Could you check a few things on this model? Use its own coordinates, in mm. A direction names the side the tool comes from. Round coordinates to 2 decimals unless told otherwise and drop trailing zeros. Loops run counter-clockwise (first coordinate to the right, second up) from the corner with the lowest first, then second, coordinate; pieces in that order, holes last. Notation, with made-up numbers: (58, 9.5) -> (73, 9.5) arc R26 ccw to (73, 43.5) -> close; hole circle Ø3 at (68.5, 48.5). An arc over 180 degrees is marked (long way). Write each question's results on one line, items separated by ' | '.
from build123d import *

# Parameters (mm, degrees)
BOSS_EXTRUDE2_DEPTH = 15
SKETCH4_R           = 2
CUT_EXTRUDE1_DEPTH  = 1
SKETCH5_R           = 1.5
BOSS_EXTRUDE3_DEPTH = 0.5
SKETCH7_W           = 3
SKETCH7_H           = 3.5
CUT_EXTRUDE2_DEPTH  = 6
LPATTERN1_COUNT     = 3
LPATTERN1_PITCH     = 5.08
SKETCH8_W           = 1
SKETCH8_H           = 6.7
BOSS_EXTRUDE4_DEPTH = 0.8
SKETCH9_W           = 1
SKETCH9_H           = 6.7
CUT_EXTRUDE3_DEPTH  = 0.8


with BuildPart() as part:
    # Sketch3 → Boss-Extrude2 (new body)
    with BuildSketch(Plane(origin=(0, 0, 0), x_dir=(0, 0, -1), z_dir=(1, 0, 0))):
        with BuildLine():
            Line((-5.15, 0), (5.15, 0))
            Line((5.15, 0), (5.15, 5.1))
            Line((5.15, 5.1), (2.75, 14.1))
            Line((2.75, 14.1), (-3.35, 14.1))
            Line((-3.35, 14.1), (-4.15, 7.7))
            ThreePointArc((-4.15, 7.7), (-4.857106781, 7.407106781), (-5.15, 6.7))
            Line((-5.15, 6.7), (-5.15, 0))
        make_face()
    extrude(amount=BOSS_EXTRUDE2_DEPTH)

    # Sketch4 → Cut-Extrude1 (cut)
    with BuildSketch(Plane(origin=(0, 14.1, 0), x_dir=(1, 0, 0), z_dir=(0, 1, 0))):
        with Locations(Location((7.5, -0.3, 0), (0, 0, 270))):
            Circle(SKETCH4_R)
    cut_extrude1 = extrude(amount=-CUT_EXTRUDE1_DEPTH, mode=Mode.SUBTRACT)

    # Sketch5 → Boss-Extrude3 (add)
    with BuildSketch(Plane(origin=(0, 13.1, 0), x_dir=(1, 0, 0), z_dir=(0, 1, 0))):
        with Locations(Location((7.5, -0.3, 0), (0, 0, 270))):
            Circle(SKETCH5_R)
    boss_extrude3 = extrude(amount=BOSS_EXTRUDE3_DEPTH)

    # Sketch-Pattern1: Cut-Extrude1, Boss-Extrude3 at 2 more places
    with Locations((5.08, 0, 0), (-5.08, 0, 0)):
        add(cut_extrude1, mode=Mode.SUBTRACT)
        add(boss_extrude3)

    # Sketch7 → Cut-Extrude2 (cut)
    with BuildSketch(Plane.XY.offset(5.15)):
        with Locations((12.58, 3.35)):
            Rectangle(SKETCH7_W, SKETCH7_H)
    cut_extrude2 = extrude(amount=-CUT_EXTRUDE2_DEPTH, mode=Mode.SUBTRACT)

    # LPattern1: Cut-Extrude2 ×3
    with Locations(*[(-i * LPATTERN1_PITCH, 0, 0) for i in range(1, LPATTERN1_COUNT)]):
        add(cut_extrude2, mode=Mode.SUBTRACT)

    # Sketch8 → Boss-Extrude4 (add)
    with BuildSketch(Plane.ZY):
        with Locations((3.65, 3.35)):
            Rectangle(SKETCH8_W, SKETCH8_H)
        with Locations((-3.15, 3.35)):
            Rectangle(SKETCH8_W, SKETCH8_H)
    extrude(amount=BOSS_EXTRUDE4_DEPTH)

    # Sketch9 → Cut-Extrude3 (cut)
    with BuildSketch(Plane(origin=(15, 0, 0), x_dir=(0, 0, -1), z_dir=(1, 0, 0))):
        with Locations((3.15, 3.35)):
            Rectangle(SKETCH9_W, SKETCH9_H)
        with Locations((-3.65, 3.35)):
            Rectangle(SKETCH9_W, SKETCH9_H)
    extrude(amount=-CUT_EXTRUDE3_DEPTH, mode=Mode.SUBTRACT)


solid = part.part
1) I'm going to push flat-ended pins straight in: pin 1 (1.2 mm diameter, centred on x = 2, z = 0.5, fed in from +Y); pin 2 (5 mm diameter, centred on x = 10.5, y = 9.5, fed in from -Z); pin 3 (3 mm diameter, centred on y = 6, z = 1.5, fed in from -X). Where does each tip first touch, or does it pass through?
Model answer:
pin 1: stops at y = 13.6 | pin 2: stops at z = -4.64 | pin 3: stops at x = 0
2) I want a section at B-B, the plane x = 2.42. Write out the boundary of the cut face in (y, z).
Model answer:
outline: (0, -5.15) -> (5.1, -5.15) -> (14.1, -2.75) -> (14.1, -1.7) -> (13.1, -1.7) -> (13.1, -1.2) -> (13.6, -1.2) -> (13.6, 1.8) -> (13.1, 1.8) -> (13.1, 2.3) -> (14.1, 2.3) -> (14.1, 3.35) -> (7.7, 4.15) arc R1 ccw to (6.7, 5.15) -> (5.1, 5.15) -> (5.1, -0.85) -> (1.6, -0.85) -> (1.6, 5.15) -> (0, 5.15) -> close
3) For faces 1 (the flat face through (7, 14.1, -2)), 2 (the flat face through (14.6, 3.3, 4.15)), 3 (the cylindrical face through (14.067, 13.346, 0.105)), 4 (the flat face through (3.92, 3, 2)), which set-ups out of +Z, -Z, +X, -X, +Y, -Y let a thin tool reach every point of the face, with its end or its side?
Model answer:
face 1: +Z, -Z, +X, -X, +Y | face 2: +X, -Y | face 3: +Y | face 4: +Z
4) I need wall thicknesses on line 1 (X direction, y = 13.95, z = 0.3); line 2 (X direction, y = 1.75, z = -0.25); line 3 (Z direction, x = 14.5, y = 4.5). Which ranges of each line are inside material? Lowest first, please.
Model answer:
line 1: x = 0 to 0.42, 4.42 to 5.5, 9.5 to 10.58, 14.58 to 15 | line 2: x = 0 to 0.92, 3.92 to 6, 9 to 11.08, 14.08 to 15 | line 3: z = -5.15 to -3.65, -2.65 to 3.15, 4.15 to 5.15
5) I want a section at A-A, the plane z = 3.75. Write out the boundary of the cut face in (x, y).
Model answer:
outline: (-0.8, 0) -> (14.2, 0) -> (14.2, 6.7) -> (15, 6.7) -> (15, 10.9) -> (0, 10.9) -> (0, 6.7) -> (-0.8, 6.7) -> close; hole (0.92, 1.6) -> (3.92, 1.6) -> (3.92, 5.1) -> (0.92, 5.1) -> close; hole (6, 1.6) -> (9, 1.6) -> (9, 5.1) -> (6, 5.1) -> close; hole (11.08, 1.6) -> (14.08, 1.6) -> (14.08, 5.1) -> (11.08, 5.1) -> close
6) I want a section at C-C, the plane y = 6.25. Write out the boundary of the cut face in (x, z).
Model answer:
outline: (-0.8, -3.65) -> (0, -3.65) -> (0, -4.84) -> (15, -4.84) -> (15, -3.65) -> (14.2, -3.65) -> (14.2, -2.65) -> (15, -2.65) -> (15, 3.15) -> (14.2, 3.15) -> (14.2, 4.15) -> (15, 4.15) -> (15, 5.15) -> (0, 5.15) -> (0, 4.15) -> (-0.8, 4.15) -> (-0.8, 3.15) -> (0, 3.15) -> (0, -2.65) -> (-0.8, -2.65) -> close
7) I want a section at D-D, the plane x = 5.25. Write out the boundary of the cut face in (y, z), plus the area to 3 significant figures.
Model answer:
outline: (0, -5.15) -> (5.1, -5.15) -> (14.1, -2.75) -> (14.1, 3.35) -> (7.7, 4.15) arc R1 ccw to (6.7, 5.15) -> (0, 5.15) -> close | area: 125 mm2
8) If we mould it in two halves opening along X, with no side actions, what happens to faces 5 (the flat face through (11.08, 3, 2)), 6 (the flat face through (7.395, 9.537, -3.967)), 7 (the flat face through (-0.8, 3, 4))? For each: released by +X, released by -X, zero draft, split by the parting line, or undercut.
Model answer:
face 5: undercut | face 6: zero draft | face 7: released by -X
